Design review of the part built by this model. Coordinates are the model's own, in mm. A direction names the side the tool comes from. Coordinates: 2 decimals unless noted, no trailing zeros. Loops run counter-clockwise (first coordinate to the right, second up) from the corner with the lowest first, then second, coordinate; pieces in that order, holes last. Notation, with made-up numbers: (11, -38) - (25, -38) arc R27 ccw to (25, -10) - close; hole circle Ø3 at (54.25, 29). An arc over 180 degrees is marked (long way). Use one line per item in the form item = value. Start each with the question number.
(1) The part is to be moulded in two halves that separate along X. For faces 3 (the face through (5, -18, -9)), 4 (the face through (-1.5, -8.4, 11.4)), 5 (the face through (-0.29, -1.48, 2.23)), say which applies: pulls with the +X half, pulls with the -X half, needs draft (parallel to the pull), parting line crosses it, or undercut.
(2) For L1, parallel to Z at x = 0, y = -0.7; L2, parallel to Y at x = -4.5, z = 1; L3, parallel to Z at x = 0, y = -11.75, list the stretches that pass through material, from the lowest coordinate up.
(3) Add section D-D (y = -2.25). State the section outline as (x, z) points, plus the area to 3 significant figures.
(4) Add section A-A (x = 0). State the section outline as (y, z) points, plus the area to 3 significant figures.
(5) Add section B-B (z = 0). State the section outline as (x, y) points, plus the area to 3 significant figures.
(6) Add section C-C (y = -6.75). State the section outline as (x, z) points.
(7) Tool access review of faces 1 (the face through (-1.172, -9.902, 8.923)), 2 (the face through (-0.2, 0, -2.4)): name each direction out of +Z, -Z, +X, -X, +Y, -Y from which nothing blocks a thin tool from reaching the whole face with its end or side.
(8) Clearance check with flat-ended pins moving along their axes: pin 1 Ø8 at (y, z) = (-2.5, 4.5) entering from -X; pin 2 Ø1 at (y, z) = (-15.5, -1.5) entering from +X; pin 3 Ø5.5 at (x, z) = (4.5, -4) entering from -Y. State where each tip first meets the part, or that it passes through.
```python
from build123d import *

# Parameters (mm, degrees)
F0_R     = 9
F0_R_2   = 2.25
F1_DEPTH = 3
F0_R_3   = 11.5
F2_DEPTH = 18
F3_R     = 1


with BuildPart() as f1:
    # F0 (on Front) → F1 (new body)
    with BuildSketch(Plane.XZ):
        Circle(F0_R)
        Circle(F0_R_2, mode=Mode.SUBTRACT)
    extrude(amount=F1_DEPTH)

    # F0 (on Front) → F2 (join)
    with BuildSketch(Plane.XZ):
        Circle(F0_R_3)
        Circle(F0_R, mode=Mode.SUBTRACT)
    extrude(amount=F2_DEPTH)

    # F3
    f3_edges = [f1.edges().sort_by_distance(p)[0] for p in [
        (-9, -18, 0),
        (-11.5, -18, 0),
    ]]
    fillet(f3_edges, radius=F3_R)


solid = f1.part
```
Computed values:
q1.face_3 = needs draft
q1.face_4 = parting line crosses it
q1.face_5 = undercut
q2.L1 = -11.5 to -2.25, 2.25 to 11.5
q2.L2 = -3 to 0
q2.L3 = -11.5 to -9, 9 to 11.5
q3.outline = circle Ø23 at (0, 0); hole circle Ø4.5 at (0, 0)
q3.area = 400 mm^2
q4.outline = (-18, -10.5) arc R1 ccw to (-17, -11.5) - (0, -11.5) - (0, -2.25) - (-3, -2.25) - (-3, -9) - (-17, -9) arc R1 ccw to (-18, -10) - close; (-18, 10) arc R1 ccw to (-17, 9) - (-3, 9) - (-3, 2.25) - (0, 2.25) - (0, 11.5) - (-17, 11.5) arc R1 ccw to (-18, 10.5) - close
q4.area = 130 mm^2
q5.outline = (-11.5, -17) arc R1 ccw to (-10.5, -18) - (-10, -18) arc R1 ccw to (-9, -17) - (-9, -3) - (-2.25, -3) - (-2.25, 0) - (-11.5, 0) - close; (2.25, -3) - (9, -3) - (9, -17) arc R1 ccw to (10, -18) - (10.5, -18) arc R1 ccw to (11.5, -17) - (11.5, 0) - (2.25, 0) - close
q5.area = 130 mm^2
q6.outline = circle Ø23 at (0, 0); hole circle Ø18 at (0, 0)
q7.face_1 = -Y
q7.face_2 = +Z, -Z, +X, -X, +Y
q8.pin_1 = -11.49
q8.pin_2 = 11.46
q8.pin_3 = -3
